Could you check a few things on this drawing? It's one solid part, dimensions in mm from its lowest x, y, z. Give positions to 0.01 mm unless a question says otherwise; leave off trailing zeros. Loops run counter-clockwise (first coordinate to the right, second up) from the corner with the lowest first, then second, coordinate; pieces in that order, holes last. Notation, with made-up numbers: (82.25, -4.5) -> (107.25, -4.5) arc R22 ccw to (107.25, 5.5) -> close; hole circle Ø9 at (-8, 22). An arc over 180 degrees is marked (long way). Use CSV: the item, a comma, the result in double quotes.
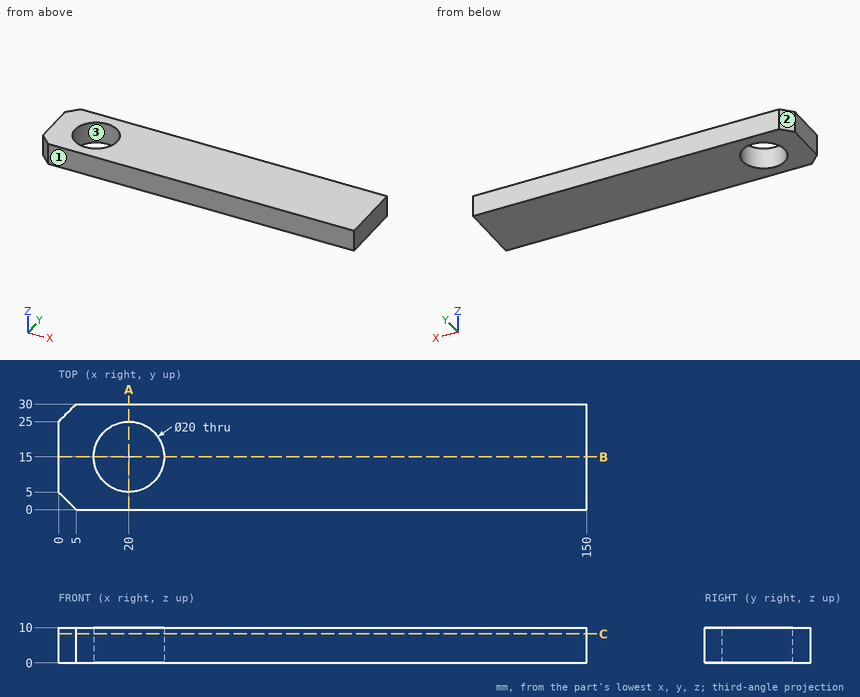
(1) If we section it at C-C, the plane z = 8.25: Write out the boundary of the cut face in (x, y), then the cut area to 3 significant figures.
Answer sheet:
outline,"(0, 5) -> (5, 0) -> (150, 0) -> (150, 30) -> (5, 30) -> (0, 25) -> close; hole circle Ø20 at (20, 15)"
area,"4,160 mm2"
(2) If we section it at B-B, the plane y = 15: Write out the boundary of the cut face in (x, z).
Answer sheet:
outline,"(0, 0) -> (10, 0) -> (10, 10) -> (0, 10) -> close; (30, 0) -> (150, 0) -> (150, 10) -> (30, 10) -> close"
(3) If we section it at A-A, the plane x = 20: Write out the boundary of the cut face in (y, z), then the cut area to 3 significant figures.
Answer sheet:
outline,"(0, 0) -> (5, 0) -> (5, 10) -> (0, 10) -> close; (25, 0) -> (30, 0) -> (30, 10) -> (25, 10) -> close"
area,"100 mm2"
(4) Will this pin go through, and if not, where does the flat tip stop? pin 1 Ø6 at (x, y) = (35, 4) entering from -Z.
Answer sheet:
pin 1,"stops at z = 0"
(5) If I drill on L1, parallel to Y at x = 20, z = 7.25; L2, parallel to Y at x = 16, z = 3; L3, parallel to X at y = 11.25, z = 9.75, over which ranges is the centre line in solid material (lowest first)? Write a range as from..to.
Answer sheet:
L1,"y = 0..5, 25..30"
L2,"y = 0..5.83, 24.17..30"
L3,"x = 0..10.73, 29.27..150"
(6) We'd pull the mould along X, two halves only. Please class the marked faces 1, 2 and 3: released by +X, released by -X, zero draft, split by the parting line, or undercut.
Answer sheet:
face 1,"zero draft"
face 2,"released by -X"
face 3,"undercut"
